Input: part model. Units: mm. Frame: model coordinates. Face numbers are marked on the shaded views. A direction names the side the tool comes from. Round coordinates to 2 decimals unless told otherwise and drop trailing zeros. Loops run counter-clockwise (first coordinate to the right, second up) from the corner with the lowest first, then second, coordinate; pieces in that order, holes last.
1) Section C-C, the plane z = -63.5. Return loops of the section in (x, y), and give its area (3 significant figures).
2) Ray query, line 1 along Y through (x, z) = (788, 119); line 2 along Y through (x, z) = (120, 115); line 3 along Z through (x, y) = (-232, -100.5). Return the intervals inside material, ascending.
3) First-contact query: pin 1 (17.5 mm diameter, centred on x = 120, y = 75, fed in from +Z); pin 2 (12 mm diameter, centred on x = -443, z = 97.5, fed in from +Y) (3 decimals); pin 3 (4 mm diameter, centred on x = 617.5, z = 75.5, fed in from -Y). Flat tips, straight axial feed; report the tip coordinate or a pass-through.
4) Section A-A, the plane y = 46.5. Return loops of the section in (x, z), and give its area (4 significant figures).
5) Access query for the marked faces 1 and 2. Directions: +Z, -Z, +X, -X, +Y, -Y. A direction counts if a zero-diameter tool reaches every point of the face in a straight line with its end or side. Return the directions, or none.
6) Draft query along Z for the marked faces 3, 4 and 5. Return one class per face: pulls with the +Z half, pulls with the -Z half, needs draft (parallel to the pull), parting line crosses it, or undercut.
7) Section B-B, the plane x = 215. Return loops of the section in (y, z).
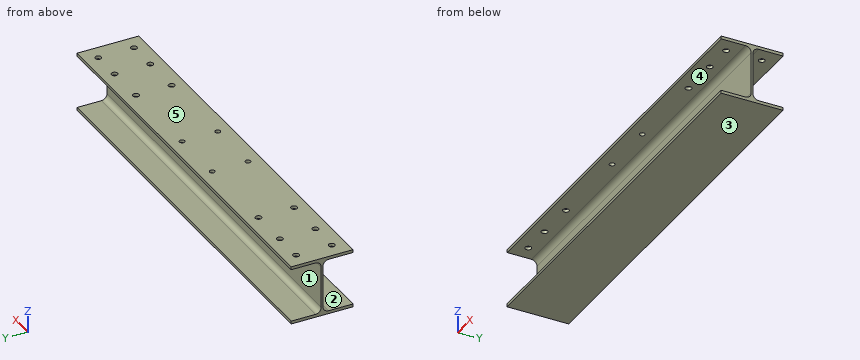
from build123d import *

# Parameters (mm, degrees)
STRUKTURBAUTEIL1_DEPTH          = 1706
SKIZZE2_R                       = 13
SKIZZE2_R_2                     = 11
SCHNITT_LINEAR_AUSTRAGEN1_DEPTH = 12.5


with BuildPart() as part:
    # Skizze12 → Strukturbauteil1 (new body)
    with BuildSketch(Plane(origin=(853, 0, 0), x_dir=(0, -1, 0), z_dir=(-1, 0, 0))):
        with BuildLine():
            Line((130, 125), (-130, 125))
            Line((-130, 125), (-130, 112.5))
            Line((-130, 112.5), (-27.75, 112.5))
            ThreePointArc((-27.75, 112.5), (-10.779437252, 105.470562748), (-3.75, 88.5))
            Line((-3.75, 88.5), (-3.75, -88.5))
            ThreePointArc((-3.75, -88.5), (-10.779437252, -105.470562748), (-27.75, -112.5))
            Line((-27.75, -112.5), (-130, -112.5))
            Line((-130, -112.5), (-130, -125))
            Line((-130, -125), (130, -125))
            Line((130, -125), (130, -112.5))
            Line((130, -112.5), (27.75, -112.5))
            ThreePointArc((27.75, -112.5), (10.779437252, -105.470562748), (3.75, -88.5))
            Line((3.75, -88.5), (3.75, 88.5))
            ThreePointArc((3.75, 88.5), (10.779437252, 105.470562748), (27.75, 112.5))
            Line((27.75, 112.5), (130, 112.5))
            Line((130, 112.5), (130, 125))
        make_face()
    extrude(amount=STRUKTURBAUTEIL1_DEPTH)

    # Skizze2 → Schnitt-Linear austragen1 (cut)
    with BuildSketch(Plane.XY.offset(125)):
        with Locations((-788, 75)):
            Circle(SKIZZE2_R)
        with Locations((-788, -75)):
            Circle(SKIZZE2_R)
        with Locations((-658, -75)):
            Circle(SKIZZE2_R)
        with Locations((-658, 75)):
            Circle(SKIZZE2_R)
        with Locations((-488, 75)):
            Circle(SKIZZE2_R)
        with Locations((-488, -75)):
            Circle(SKIZZE2_R)
        with Locations(Location((488, -75, 0), (0, 0, 270))):  # turned: the seam where the file's is
            Circle(SKIZZE2_R)
        with Locations(Location((488, 75, 0), (0, 0, 270))):  # turned: the seam where the file's is
            Circle(SKIZZE2_R)
        with Locations(Location((658, 75, 0), (0, 0, 270))):  # turned: the seam where the file's is
            Circle(SKIZZE2_R)
        with Locations(Location((658, -75, 0), (0, 0, 270))):  # turned: the seam where the file's is
            Circle(SKIZZE2_R)
        with Locations(Location((788, -75, 0), (0, 0, 270))):  # turned: the seam where the file's is
            Circle(SKIZZE2_R)
        with Locations(Location((788, 75, 0), (0, 0, 270))):  # turned: the seam where the file's is
            Circle(SKIZZE2_R)
        with Locations((-120, 75)):
            Circle(SKIZZE2_R_2)
        with Locations((120, 75)):
            Circle(SKIZZE2_R_2)
        with Locations((-120, -75)):
            Circle(SKIZZE2_R_2)
        with Locations((120, -75)):
            Circle(SKIZZE2_R_2)
    extrude(amount=-SCHNITT_LINEAR_AUSTRAGEN1_DEPTH, mode=Mode.SUBTRACT)


solid = part.part
Final values:
1. outline: (-853, -3.75) - (853, -3.75) - (853, 3.75) - (-853, 3.75) - close
1. area: 12,800 mm2
2. line 1: y = -130 to -88, -62 to 62, 88 to 130
2. line 2: y = -130 to -86, -64 to 64, 86 to 130
2. line 3: z = -125 to -112.5, 112.5 to 125
3. pin 1: stops at z = -112.5
3. pin 2: stops at y = 9.015
3. pin 3: stops at y = -3.75
4. outline: (-853, -125) - (853, -125) - (853, -112.5) - (-853, -112.5) - close; (-853, 112.5) - (853, 112.5) - (853, 125) - (-853, 125) - close
4. area: 42,650 mm2
5. face 1: +X, -X, +Y
5. face 2: +X, -X, -Y
6. face 3: pulls with the -Z half
6. face 4: undercut
6. face 5: pulls with the +Z half
7. outline: (-130, -125) - (130, -125) - (130, -112.5) - (27.75, -112.5) arc R24 cw to (3.75, -88.5) - (3.75, 88.5) arc R24 cw to (27.75, 112.5) - (130, 112.5) - (130, 125) - (-130, 125) - (-130, 112.5) - (-27.75, 112.5) arc R24 cw to (-3.75, 88.5) - (-3.75, -88.5) arc R24 cw to (-27.75, -112.5) - (-130, -112.5) - close
